Verification items for this drawing (mm, ordinates from the low corner). Coordinates: 2 decimals unless noted, no trailing zeros. Write each loop counter-clockwise with the first axis right and the second up, starting at its lowest first coordinate (ties: lowest second). Pieces come first, ordered by that corner, then holes. Notation, with made-up numbers: M 3,-36.75 L 30,-36.75 A25 cw 30,-14.75 Z; hole C -5,-3 d10. An arc over 180 degrees is marked long. Put each result on its own line as item: value. Start each with the question number.
1) Gauge pin test, flat ends, axial feed: pin 1 (12 mm diameter, centred on y = 112.63, z = 92.5, fed in from -X); pin 2 (8.5 mm diameter, centred on y = 112.63, z = 37.5, fed in from +X). Record the tip position at first contact, or that the pin passes through.
2) Cross-section at A-A on z = 65. Record the cut outline in (x, y), plus the area to 3 significant figures.
3) Cross-section at B-B on y = 65. Record the cut outline in (x, z).
4) Cross-section at D-D on x = 1.15. Count the separate pieces of the cut face and the enclosed holes in it, plus the area to 3 significant figures.
5) Cross-section at C-C on z = 37. Record the cut outline in (x, y) (1 decimal).
6) Scan lines: line 1 along Y through (x, z) = (1.4, 38) (1 decimal); line 2 along Z through (x, y) = (1.65, 21.5); line 3 along Z through (x, y) = (0.8, 21) (1 decimal). Record each from-to range of solid material in increasing order.
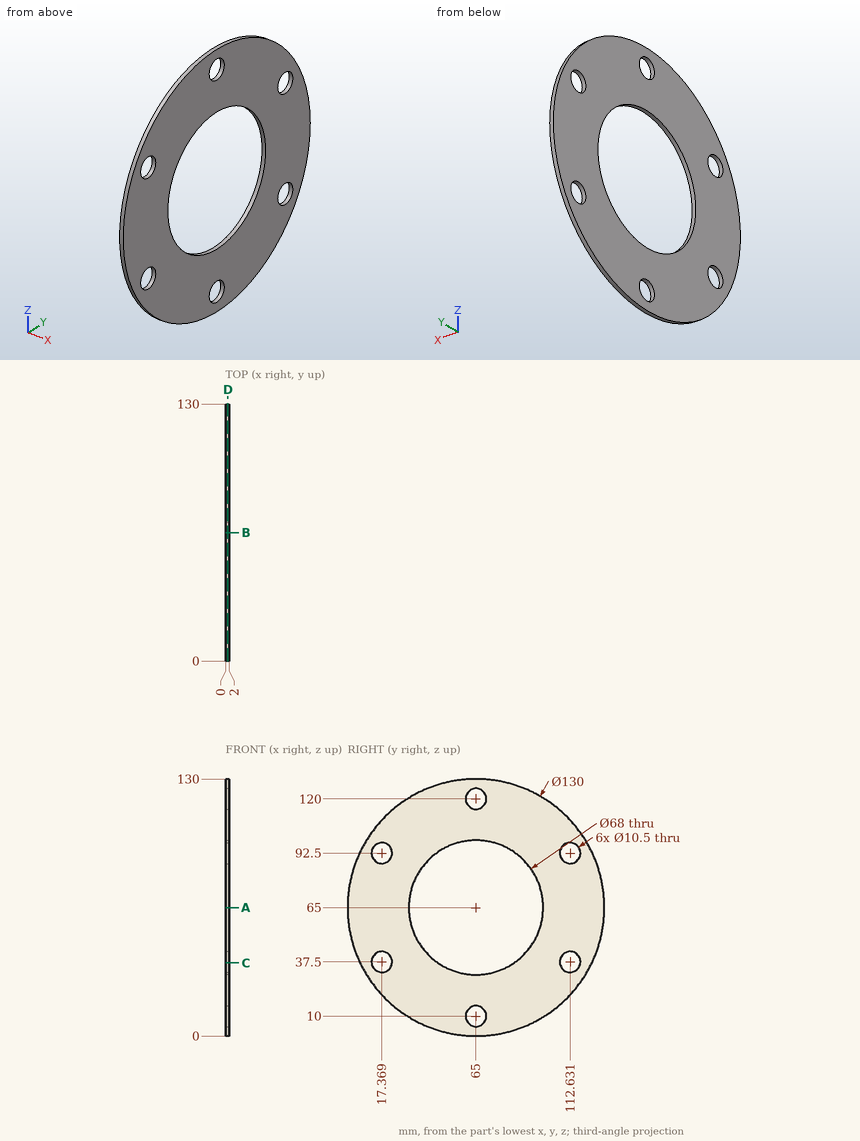
Answer key:
1. pin 1: stops at x = 0
1. pin 2: passes through
2. outline: M 0,0 L 2,0 L 2,31 L 0,31 Z; M 0,99 L 2,99 L 2,130 L 0,130 Z
2. area: 124 mm²
3. outline: M 0,0 L 2,0 L 2,4.75 L 0,4.75 Z; M 0,15.25 L 2,15.25 L 2,31 L 0,31 Z; M 0,99 L 2,99 L 2,114.75 L 0,114.75 Z; M 0,125.25 L 2,125.25 L 2,130 L 0,130 Z
4. separate pieces: 1
4. enclosed holes: 7
4. area: 9,120 mm²
5. outline: M 0,6.3 L 2,6.3 L 2,12.1 L 0,12.1 Z; M 0,22.6 L 2,22.6 L 2,45.7 L 0,45.7 Z; M 0,84.3 L 2,84.3 L 2,107.4 L 0,107.4 Z; M 0,117.9 L 2,117.9 L 2,123.7 L 0,123.7 Z
6. line 1: y = 5.9 to 12.1, 22.6 to 44.3, 85.7 to 107.4, 117.9 to 124.1
6. line 2: z = 16.7 to 34.26, 40.74 to 89.26, 95.74 to 113.3
6. line 3: z = 17.2 to 33.7, 41.3 to 88.7, 96.3 to 112.8
